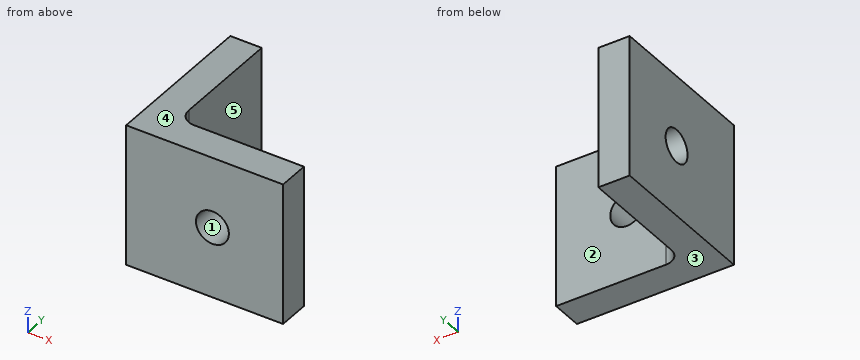
from build123d import *

# Parameters (mm, degrees)
DODANIE_WYCI_GNI_CIE1_DEPTH = 18
SZKIC2_R                    = 2.1
WYTNIJ_WYCI_GNI_CIE1_DEPTH  = 32.304951685
SZKIC3_R                    = 2.1
WYTNIJ_WYCI_GNI_CIE2_DEPTH  = 32.304951685
ZAOKR_GLENIE1_R             = 2


with BuildPart() as part:
    # Szkic1 → Dodanie-wyciągnięcie1 (new body)
    with BuildSketch(Plane.XY):
        Polygon((0, 0), (20, 0), (20, 4), (4, 4), (4, 20), (0, 20), align=None)
    extrude(amount=DODANIE_WYCI_GNI_CIE1_DEPTH)

    # Szkic2 → Wytnij-wyciągnięcie1 (cut, through all)
    with BuildSketch(Plane(origin=(4, 0, 0), x_dir=(0, 0, -1), z_dir=(1, 0, 0))):
        with Locations(Location((-9, 11, 0), (0, 0, 90))):
            Circle(SZKIC2_R)
    extrude(amount=-WYTNIJ_WYCI_GNI_CIE1_DEPTH, mode=Mode.SUBTRACT)

    # Szkic3 → Wytnij-wyciągnięcie2 (cut, through all)
    with BuildSketch(Plane(origin=(0, 4, 0), x_dir=(1, 0, 0), z_dir=(0, 1, 0))):
        with Locations(Location((11, -9, 0), (0, 0, 180))):
            Circle(SZKIC3_R)
    extrude(amount=-WYTNIJ_WYCI_GNI_CIE2_DEPTH, mode=Mode.SUBTRACT)

    # Zaokrąglenie1
    zaokr_glenie1_edges = [part.edges().sort_by_distance(p)[0] for p in [
        (4, 4, 9),
    ]]
    fillet(zaokr_glenie1_edges, radius=ZAOKR_GLENIE1_R)


solid = part.part
Read the model definition and answer for the solid it produces. Units are mm, in the model's axes. Face numbers are marked on the shaded views. A direction names the side the tool comes from. Round coordinates to 2 decimals unless told otherwise and drop trailing zeros. Loops run counter-clockwise (first coordinate to the right, second up) from the corner with the lowest first, then second, coordinate; pieces in that order, holes last.
Q1. Each of these flat-tipped pins is pushed along its axis until it touches: pin 1 (4 mm diameter, centred on x = 12.5, z = 11, fed in from +Y); pin 2 (4 mm diameter, centred on y = 13, z = 7.5, fed in from +X); pin 3 (3 mm diameter, centred on y = 7, z = 15.5, fed in from +X). Where does it stop, or does it pass through?
Q2. Section D-D on z = 12 is taken. Write down the section's boundary in (x, y).
Q3. Consider probe 1 along Z at (x, y) = (2.3, 11); probe 2 along X at (y, z) = (16.5, 3). Determine where each line is inside the solid, lowest interval first.
Q4. Determine the mould class of the marked faces 1, 2 and 3 for opening direction Z: released by +Z, released by -Z, zero draft, split by the parting line, or undercut.
Q5. Which of the six approach directions +Z, -Z, +X, -X, +Y, -Y give full straight-line access (tool end or side, diameter ignored) to the marked faces 4 and 5?
Q6. Section B-B on z = 9 is taken. Write down the section's boundary in (x, y).
Q7. Section A-A on y = 11 is taken. Write down the section's boundary in (x, z), and give its area (3 significant figures).
Output:
1. pin 1: stops at y = 4
1. pin 2: stops at x = 4
1. pin 3: stops at x = 4.06
2. outline: (0, 0) - (20, 0) - (20, 4) - (6, 4) arc R2 cw to (4, 6) - (4, 20) - (0, 20) - close
3. probe 1: z = 0 to 6.9, 11.1 to 18
3. probe 2: x = 0 to 4
4. face 1: undercut
4. face 2: zero draft
4. face 3: released by -Z
5. face 4: +Z, +X, -X, +Y, -Y
5. face 5: +Z, -Z, +X, +Y
6. outline: (0, 0) - (8.9, 0) - (8.9, 4) - (6, 4) arc R2 cw to (4, 6) - (4, 8.9) - (0, 8.9) - close; (0, 13.1) - (4, 13.1) - (4, 20) - (0, 20) - close; (13.1, 0) - (20, 0) - (20, 4) - (13.1, 4) - close
7. outline: (0, 0) - (4, 0) - (4, 6.9) - (0, 6.9) - close; (0, 11.1) - (4, 11.1) - (4, 18) - (0, 18) - close
7. area: 55.2 mm2
